from build123d import *

# Parameters (mm, degrees)
BOSS_EXTRUDE1_DEPTH = 5.5
SKETCH2_R           = 30
SKETCH2_R_2         = 17.5
SKETCH2_R_3         = 12.5
SKETCH2_R_4         = 5
BOSS_EXTRUDE2_DEPTH = 99
SKETCH3_R           = 17.5
SKETCH3_R_2         = 5
CUT_EXTRUDE1_DEPTH  = 99
SKETCH4_R           = 5
CUT_EXTRUDE2_DEPTH  = 99
SKETCH5_R           = 17.5
CUT_EXTRUDE3_DEPTH  = 99


with BuildPart() as part:
    # Sketch1 → Boss-Extrude1 (new body)
    with BuildSketch(Plane.XY):
        with BuildLine():
            Line((6.228918342, 39.512030779), (130, 20))
            ThreePointArc((130, 20), (150, 0), (130, -20))
            Line((130, -20), (6.228918342, -39.512030779))
            ThreePointArc((6.228918342, -39.512030779), (-40, 0), (6.228918342, 39.512030779))
        make_face()
    boss_extrude1 = extrude(amount=BOSS_EXTRUDE1_DEPTH)

    # Sketch2 → Boss-Extrude2 (add)
    with BuildSketch(Plane.XY.offset(20.5)):
        Circle(SKETCH2_R)
        Circle(SKETCH2_R_2, mode=Mode.SUBTRACT)
        with Locations((130, 0)):
            Circle(SKETCH2_R_3)
        with Locations((130, 0)):
            Circle(SKETCH2_R_4, mode=Mode.SUBTRACT)
    extrude(amount=-BOSS_EXTRUDE2_DEPTH)

    # Sketch3 → Cut-Extrude1 (cut)
    with BuildSketch(Plane.XY.offset(5.5)):
        Circle(SKETCH3_R)
        with Locations((130, 0)):
            Circle(SKETCH3_R_2)
    extrude(amount=-CUT_EXTRUDE1_DEPTH, mode=Mode.SUBTRACT)

    # Mirror5: Boss-Extrude1 across plane
    add(boss_extrude1.mirror(Plane.XY.offset(-27.5)))

    # Sketch4 → Cut-Extrude2 (cut)
    with BuildSketch(Plane(origin=(0, 0, -60.5), x_dir=(-1, 0, 0), z_dir=(0, 0, -1))):
        with Locations((-130, 0)):
            Circle(SKETCH4_R)
    extrude(amount=-CUT_EXTRUDE2_DEPTH, mode=Mode.SUBTRACT)

    # Sketch5 → Cut-Extrude3 (cut)
    with BuildSketch(Plane(origin=(0, 0, -60.5), x_dir=(-1, 0, 0), z_dir=(0, 0, -1))):
        Circle(SKETCH5_R)
    extrude(amount=-CUT_EXTRUDE3_DEPTH, mode=Mode.SUBTRACT)


solid = part.part
Part model, mm, in its own coordinate system. A direction names the side the tool comes from. Give positions to 0.01 mm unless a question says otherwise; leave off trailing zeros. Loops run counter-clockwise (first coordinate to the right, second up) from the corner with the lowest first, then second, coordinate; pieces in that order, holes last.
(1) Band-saw the part on A-A (x = 0). Write the cut outline in (y, z).
Return value:
outline: (-40, -60.5) - (-30, -60.5) - (-30, -78.5) - (-17.5, -78.5) - (-17.5, 20.5) - (-30, 20.5) - (-30, 5.5) - (-40, 5.5) - (-40, 0) - (-30, 0) - (-30, -55) - (-40, -55) - close; (17.5, -78.5) - (30, -78.5) - (30, -60.5) - (40, -60.5) - (40, -55) - (30, -55) - (30, 0) - (40, 0) - (40, 5.5) - (30, 5.5) - (30, 20.5) - (17.5, 20.5) - close
(2) Pin check, flat tips, straight feed: pin 1 (3 mm diameter, centred on y = -6, z = -16, fed in from +X); pin 2 (6 mm diameter, centred on y = -27.5, z = -9.5, fed in from +X); pin 3 (4 mm diameter, centred on y = -22.5, z = -57.5, fed in from -X). Stop position of each tip, or through.
Return value:
pin 1: stops at x = 141.66
pin 2: stops at x = 17.31
pin 3: stops at x = -34.35
(3) Band-saw the part on D-D (y = 28). Write the cut outline in (x, z).
Return value:
outline: (-28.57, -60.5) - (-10.77, -60.5) - (-10.77, -78.5) - (10.77, -78.5) - (10.77, -60.5) - (79.25, -60.5) - (79.25, -55) - (10.77, -55) - (10.77, 0) - (79.25, 0) - (79.25, 5.5) - (10.77, 5.5) - (10.77, 20.5) - (-10.77, 20.5) - (-10.77, 5.5) - (-28.57, 5.5) - (-28.57, 0) - (-10.77, 0) - (-10.77, -55) - (-28.57, -55) - close
(4) Drill centre lines: line 1 along Z through (x, y) = (82.5, 16); line 2 along Y through (x, z) = (0, -59.35); line 3 along Y through (x, z) = (130, -58). Where is each one in solid material? Low to high.
Return value:
line 1: z = -60.5 to -55, 0 to 5.5
line 2: y = -40 to -17.5, 17.5 to 40
line 3: y = -20 to -5, 5 to 20
(5) Band-saw the part on C-C (z = -3). Write the cut outline in (x, y), and give its area (3 significant figures).
Return value:
outline: circle Ø60 at (0, 0); circle Ø25 at (130, 0); hole circle Ø35 at (0, 0); hole circle Ø10 at (130, 0)
area: 2,280 mm2
(6) Band-saw the part on B-B (y = -33.5). Write the cut outline in (x, z).
Return value:
outline: (-21.86, -60.5) - (44.37, -60.5) - (44.37, -55) - (-21.86, -55) - close; (-21.86, 0) - (44.37, 0) - (44.37, 5.5) - (-21.86, 5.5) - close
(7) Pull direction X, two halves, no side cores. Call faces 1 (the flat face through (56, 1, -60.5)), 2 (the flat face through (67.2, 29.9, -57.7)), 3 (the flat face through (13, -13, -78.5)): pulls with the +X half, pulls with the -X half, needs draft (parallel to the pull), parting line crosses it, or undercut.
Return value:
face 1: undercut
face 2: pulls with the +X half
face 3: needs draft
(8) 3-axis set-ups, long thin cutter, end or side, ignore diameter. For faces 4 (the flat face through (56, 1, 5.5)), 5 (the cylindrical face through (-29.97, 1.32, -27.11)), 6 (the cylindrical face through (-29.97, 1.32, -69.37)): which of +Z, -Z, +X, -X, +Y, -Y reach the whole face in a straight line?
Return value:
face 4: +Z
face 5: none
face 6: -Z
